Autodesk Inventor part; units mm, degrees
ref_plane "YZ Plane" through (0, 0, 0) normal (1, 0, 0) x (0, 1, 0)
ref_plane "XZ Plane" through (0, 0, 0) normal (0, 1, 0) x (-1, 0, 0)
ref_plane "XY Plane" through (0, 0, 0) normal (0, 0, 1) x (1, 0, 0)
sketch "Sketch1" plane through (0, 0, 0) normal (0, 1, 0) x (-1, 0, 0)
  line L0 (6.35, 0) -> (69.85, 0)
  line L1 (76.2, -6.35) -> (76.2, -69.85)
  line L2 (69.85, -76.2) -> (6.35, -76.2)
  line L3 (0, -69.85) -> (0, -6.35)
  line L4 (69.85, 0) -> (76.2, -6.35)
  line L5 (76.2, -69.85) -> (69.85, -76.2)
  line L6 (6.35, 0) -> (0, -6.35)
  line L7 (6.35, -76.2) -> (0, -69.85)
  point P0 (0, 0)
  point P1 (76.2, -76.2)
  point P2 (76.2, 0)
  point P3 (0, -76.2)
  dimension "d2" = 76.2
  dimension "d3" = 76.2
  dimension "d4" = 6.35
  dimension "d5" = 6.35
  dimension "d6" = 6.35
  dimension "d7" = 6.35
  dimension "d8" = 6.35
  dimension "d9" = 6.35
  dimension "d10" = 6.35
  dimension "d11" = 6.35
extrude "Extrusion1" add sketch "Sketch1" along normal blind 101.6
sketch "Sketch2" plane through (0, 101.6, 0) normal (0, 1, 0) x (1, 0, 0)
  circle A0 centre (-38.1, 38.1) radius 19.05
  line L0 (-69.85, 0) -> (-6.35, 0)
  line L1 (0, 6.35) -> (0, 69.85)
  point P0 (0, 0)
  dimension "d14" = 38.1
  dimension "d15" = 38.1
  dimension "d16" = 38.1
extrude "Extrusion2" add sketch "Sketch2" along normal blind 12.7
sketch "Sketch3" plane through (-38.1, 114.3, -38.1) normal (0, 1, 0) x (1, 0, 0)
  circle A0 centre (0, 0) radius 50.8
  point P0 (38.1, -38.1)
  dimension "d19" = 101.6
extrude "Extrusion3" add sketch "Sketch3" along normal blind 25.4
properties part number "Motor"
Build history of the part. All positions in model axes, mm. A direction names the side the tool comes from. Coordinates: 2 decimals unless noted, no trailing zeros. Order: outer loops, then holes, each group sorted by start corner. A loop starts at its lowest first (then second) coordinate and runs counter-clockwise, first axis right, second up. Notation, with made-up numbers: M -18,10 L -13,10 A20 cw -13,21 Z; hole C 7.5,42.5 d9. An arc over 180 degrees is marked long. One line per question, with ' | ' between items. Start each with the question number.
Q1. Saw through at A-A (x = -72.5). List the corners of the cut face in (y, z).
Q2. Saw through at D-D (y = 11). List the corners of the cut face in (x, z), then the cut area to 3 significant figures.
Q3. Probe L1, parallel to Y at x = -40, z = -13.5; L2, parallel to Z at x = -67.5, y = 61. List the from-to ranges inside material, lowest first. Write a range as from..to.
Q4. Two-plate mould, pull along Y, no slides. Class faces 1 (the face through (-21, 101.6, -29)), 2 (the face through (-3.22, 50.09, -3.13)), 3 (the face through (-38, 0, -38)): +Y half, -Y half, draft (parallel to the pull), parting line (faces both ways), or undercut.
Q5. Saw through at B-B (z = -10). List the corners of the cut face in (x, y).
Q6. Flat gauge pins, fed straight in: pin 1 Ø19 at (x, y) = (-50, 68.5) entering from -Z; pin 2 Ø3 at (x, y) = (-29.5, 108) entering from +Z; pin 3 Ø10 at (x, y) = (-46.5, 116.5) entering from +Z; pin 4 Ø3 at (x, z) = (-50, -31) entering from -Y. Where does each tip first touch, or does it go through?
Q7. Saw through at C-C (x = -38.1). List the corners of the cut face in (y, z).
Q8. 3-axis set-ups, long thin cutter, end or side, ignore diameter. For faces 4 (the face through (-27.859, 107.861, -22.037)), 5 (the face through (-76.2, 50, -38)), 6 (the face through (-39, 50, -76.2)), 7 (the face through (0, 50, -39)): which of +Z, -Z, +X, -X, +Y, -Y reach the whole face in a straight line?
Check values:
1) outline: M 0,-73.55 L 101.6,-73.55 L 101.6,-2.65 L 0,-2.65 Z; M 114.3,-75.48 L 139.7,-75.48 L 139.7,-0.72 L 114.3,-0.72 Z
2) outline: M -76.2,-69.85 L -69.85,-76.2 L -6.35,-76.2 L 0,-69.85 L 0,-6.35 L -6.35,0 L -69.85,0 L -76.2,-6.35 Z | area: 5,730 mm2
3) L1: y = 0..101.6, 114.3..139.7 | L2: z = -76.2..0
4) face 1: undercut | face 2: draft | face 3: -Y half
5) outline: M -80.42,114.3 L 4.22,114.3 L 4.22,139.7 L -80.42,139.7 Z; M -76.2,0 L 0,0 L 0,101.6 L -76.2,101.6 Z
6) pin 1: stops at z = -76.2 | pin 2: stops at z = -20.42 | pin 3: stops at z = 12.59 | pin 4: stops at y = 0
7) outline: M 0,-76.2 L 101.6,-76.2 L 101.6,-57.15 L 114.3,-57.15 L 114.3,-88.9 L 139.7,-88.9 L 139.7,12.7 L 114.3,12.7 L 114.3,-19.05 L 101.6,-19.05 L 101.6,0 L 0,0 Z
8) face 4: none | face 5: +Z, -Z, -X, -Y | face 6: -Z, +X, -X, -Y | face 7: +Z, -Z, +X, -Y
